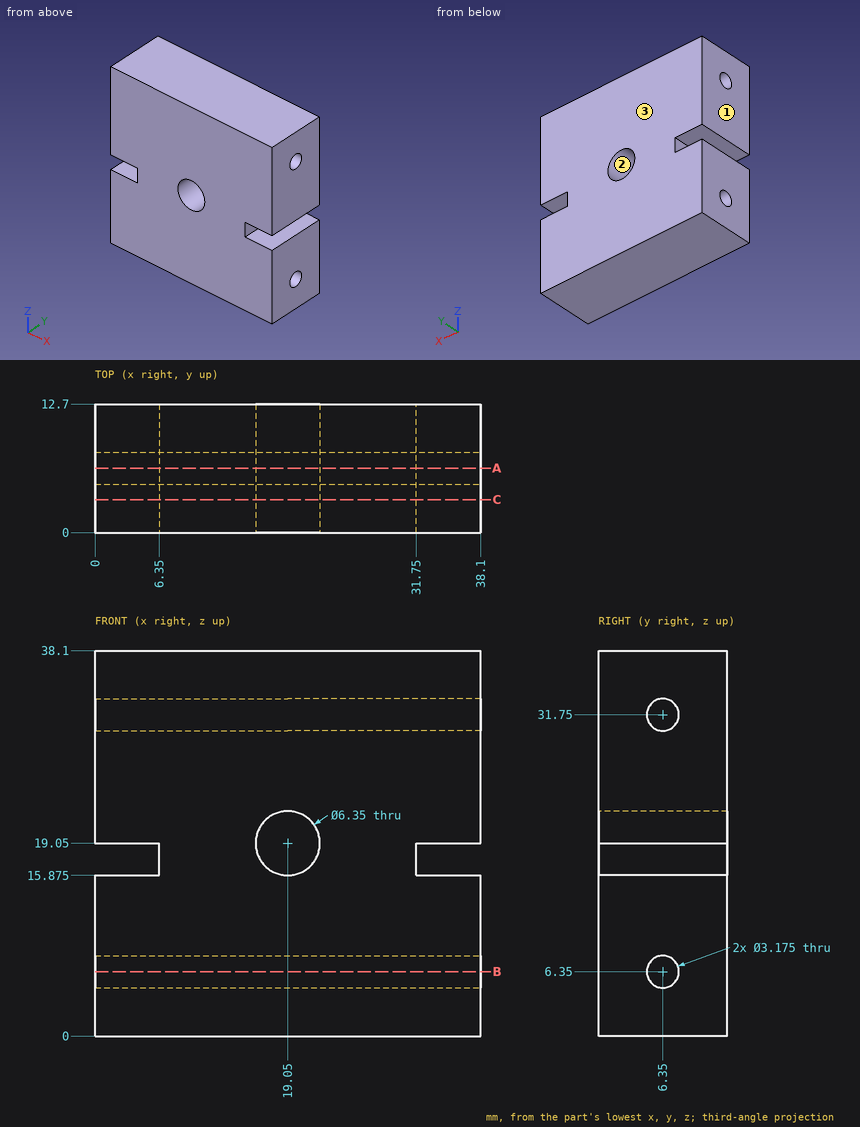
Study the drawing (mm; zero at the part's minimum x, y, z) and answer. Give positions to 0.01 mm unless a question says otherwise; leave off trailing zeros. Order: outer loops, then holes, each group sorted by start corner. A loop starts at its lowest first (then second) coordinate and runs counter-clockwise, first axis right, second up. Notation, with made-up numbers: M 66.5,23 L 116.5,23 A25 cw 116.5,48 Z; hole C 62,88.25 d8. An arc over 180 degrees is marked long. Put each result on its own line as item: value. Start each with the question number.
Item 1: Find the intervals of material crossed by line 1 along Z through (x, y) = (13.5, 6.5); line 2 along Z through (x, y) = (19.05, 3) (3 decimals); line 3 along Z through (x, y) = (20, 6.35), in increasing order.
Item 2: A flat-ended cylindrical pin translates along its axis: P1, Ø1.6, axis at y = 6, z = 18, coming from the -X side. Find the tip coordinate at first contact, or state that the pin passes through.
Item 3: The part is cut by section A-A, the plane y = 6.35. State how many separate pieces and enclosed holes the cut face has, and give its area (3 significant figures).
Item 4: The part is cut by section C-C, the plane y = 3.25. Determine the outline of the cut face in (x, z) (3 decimals).
Item 5: The part is cut by section B-B, the plane z = 6.35. Determine the outline of the cut face in (x, y).
Item 6: For a pull along X with two mould halves and no side action, classify the marked faces 1, 2 and 3 as +X half, -X half, draft (parallel to the pull), parting line (faces both ways), or undercut.
Answer key:
1. line 1: z = 0 to 4.77, 7.93 to 30.17, 33.33 to 38.1
1. line 2: z = 0 to 15.875, 22.225 to 38.1
1. line 3: z = 0 to 4.76, 7.94 to 16.02, 22.08 to 30.16, 33.34 to 38.1
2. P1: stops at x = 6.35
3. separate pieces: 3
3. enclosed holes: 1
3. area: 1,140 mm²
4. outline: M 0,0 L 38.1,0 L 38.1,15.875 L 31.75,15.875 L 31.75,19.05 L 38.1,19.05 L 38.1,38.1 L 0,38.1 L 0,19.05 L 6.35,19.05 L 6.35,15.875 L 0,15.875 Z; hole C 19.05,19.05 d6.35
5. outline: M 0,0 L 38.1,0 L 38.1,4.76 L 0,4.76 Z; M 0,7.94 L 38.1,7.94 L 38.1,12.7 L 0,12.7 Z
6. face 1: -X half
6. face 2: undercut
6. face 3: draft
